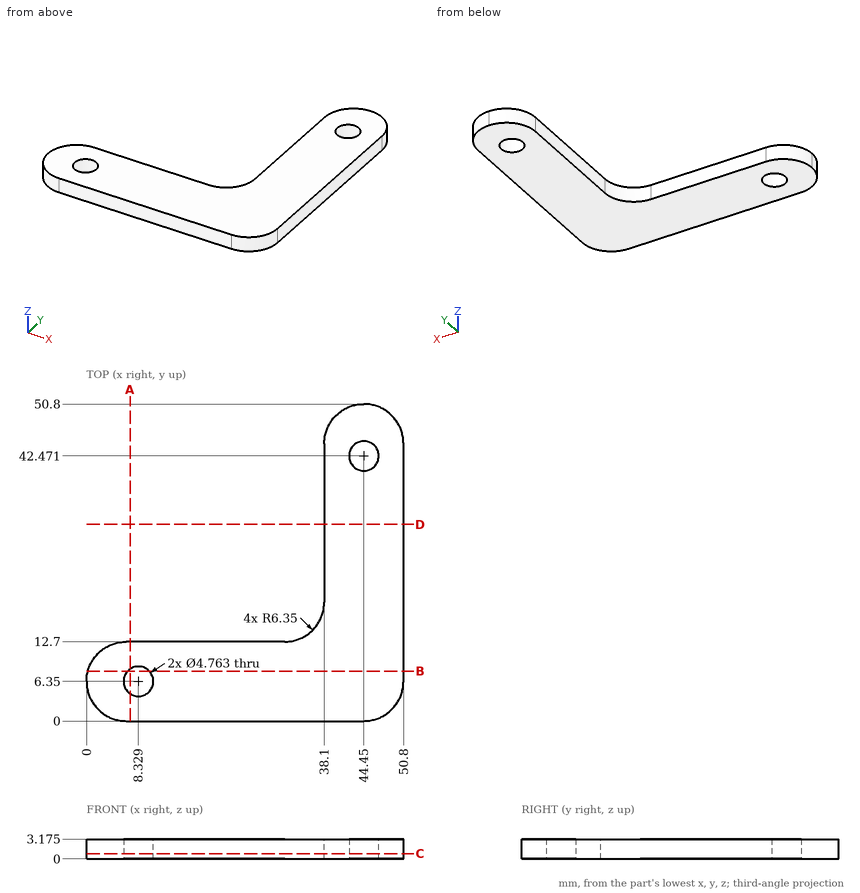
Answer from the drawing. Dimensions are ordinates in mm from the lowest x, y and z of the part. Coordinates: 2 decimals unless noted, no trailing zeros. Write each loop counter-clockwise with the first axis right and the second up, starting at its lowest first coordinate (ties: lowest second). Pieces come first, ordered by that corner, then holes. Notation, with made-up numbers: M 16.5,47 L 47.5,47 A19 ccw 47.5,68 Z; hole C 56.25,40 d9. An arc over 180 degrees is marked long. Put each result on its own line as item: value. Start each with the question number.
1. Consider line 1 (Y direction, x = 44.45, z = 1.6); line 2 (Y direction, x = 14, z = 1.5); line 3 (Y direction, x = 6.5, z = 1.3) (1 decimal). Determine where each line is inside the solid, lowest interval first. Write a range as from..to.
2. A cutting plane is placed at C-C on z = 0.85. Count the separate pieces of the cut face and the enclosed holes in it, then the cut area to 3 significant figures.
3. A cutting plane is placed at A-A on x = 7. Write down the section's boundary in (y, z) (1 decimal).
4. A cutting plane is placed at B-B on y = 8. Write down the section's boundary in (x, z) (1 decimal).
5. Flat-ended cylindrical pins translate along their axes: P1, Ø1.5, axis at y = 26, z = 0.5, coming from the -X side; P2, Ø1.6, axis at x = 15.5, z = 2, coming from the +Y side; P3, Ø1.5, axis at x = 27.5, z = 1, coming from the -Y side. Find the tip coordinate at first contact, or state that the pin passes through.
6. A cutting plane is placed at D-D on y = 31.5. Write down the section's boundary in (x, z) (1 decimal).
Resolved:
1. line 1: y = 0..40.09, 44.85..50.8
1. line 2: y = 0..12.7
1. line 3: y = 0..4.8, 7.9..12.7
2. separate pieces: 1
2. enclosed holes: 2
2. area: 1,060 mm2
3. outline: M 0,0 L 4.4,0 L 4.4,3.2 L 0,3.2 Z; M 8.3,0 L 12.7,0 L 12.7,3.2 L 8.3,3.2 Z
4. outline: M 0.2,0 L 6.6,0 L 6.6,3.2 L 0.2,3.2 Z; M 10,0 L 50.8,0 L 50.8,3.2 L 10,3.2 Z
5. P1: stops at x = 38.1
5. P2: stops at y = 12.7
5. P3: stops at y = 0
6. outline: M 38.1,0 L 50.8,0 L 50.8,3.2 L 38.1,3.2 Z
